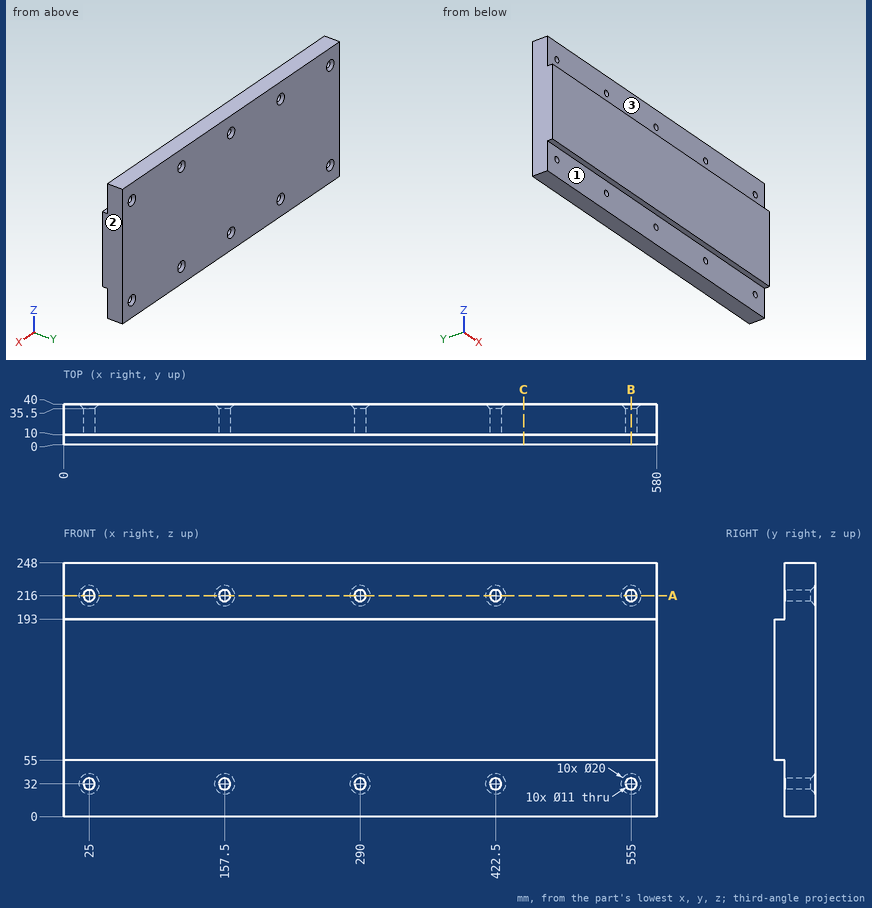
Verification items for this drawing (mm, ordinates from the low corner). A direction names the side the tool comes from. Coordinates: 2 decimals unless noted, no trailing zeros. Order: outer loops, then holes, each group sorted by start corner. A loop starts at its lowest first (then second) coordinate and runs counter-clockwise, first axis right, second up.
Q1. Sectioned sample at C-C on x = 450. Record the cut outline in (y, z), and give its area (3 significant figures).
Reply:
outline: (0, 55) - (10, 55) - (10, 0) - (40, 0) - (40, 248) - (10, 248) - (10, 193) - (0, 193) - close
area: 8,820 mm2
Q2. Sectioned sample at B-B on x = 555. Record the cut outline in (y, z), and give its area (3 significant figures).
Reply:
outline: (0, 55) - (10, 55) - (10, 37.5) - (35.5, 37.5) - (40, 42) - (40, 206) - (35.5, 210.5) - (10, 210.5) - (10, 193) - (0, 193) - close; (10, 0) - (40, 0) - (40, 22) - (35.5, 26.5) - (10, 26.5) - close; (10, 221.5) - (35.5, 221.5) - (40, 226) - (40, 248) - (10, 248) - close
area: 8,120 mm2
Q3. Sectioned sample at A-A on z = 216. Give the number of separate pieces and of enclosed holes in the cut face, and give its area (3 significant figures).
Reply:
separate pieces: 6
enclosed holes: 0
area: 15,600 mm2
Q4. Depth check by flat-ended pin: pin 1 Ø17.5 at (x, z) = (157.5, 216) entering from -Y; pin 2 Ø1 at (x, y) = (467.5, 4) entering from +Z; pin 3 Ø6.5 at (x, z) = (25, 216) entering from -Y; pin 4 Ø2 at (x, y) = (200, 6) entering from -Z. Enter the tip coordinate at first touch or a pass-through.
Reply:
pin 1: stops at y = 10
pin 2: stops at z = 193
pin 3: passes through
pin 4: stops at z = 55
Q5. Tool access check on the marked faces 1, 2 and 3. Record the directions out of +Z, -Z, +X, -X, +Y, -Y that give a thin tool (end or side, any length) a straight path to the whole face; none if there is none.
Reply:
face 1: -Z, +X, -X, -Y
face 2: +Z, -Z, +X, +Y, -Y
face 3: +Z, +X, -X, -Y
Q6. Thickness scan on probe 1 along X at (y, z) = (19.75, 32); probe 2 along Z at (x, y) = (157.5, 16); probe 3 along Y at (x, z) = (304, 50). Record the ranges inside material, lowest first.
Reply:
probe 1: x = 0 to 19.5, 30.5 to 152, 163 to 284.5, 295.5 to 417, 428 to 549.5, 560.5 to 580
probe 2: z = 0 to 26.5, 37.5 to 210.5, 221.5 to 248
probe 3: y = 10 to 40
